```python
from build123d import *

# Parameters (mm, degrees)
F2_W     = 50
F2_H     = 40
F3_DEPTH = 1.5
F4_D     = 3.5


with BuildPart() as f3:
    # F2 (on Top) → F3 (new body)
    with BuildSketch(Plane.XY):
        Rectangle(F2_W, F2_H)
    extrude(amount=F3_DEPTH)

    # F4 (through all)
    with Locations(Plane(origin=(0, 0, 0), x_dir=(1, 0, 0), z_dir=(0, 0, -1))):
        with Locations((-22.2, 17.2), (-22.2, -17.2), (22.2, 17.2), (22.2, -17.2)):
            Hole(F4_D / 2)


solid = f3.part
```
The model under review builds one solid part; all positions refer to its coordinate system, in mm. Coordinates: 2 decimals unless noted, no trailing zeros. Write each loop counter-clockwise with the first axis right and the second up, starting at its lowest first coordinate (ties: lowest second). Pieces come first, ordered by that corner, then holes. Notation, with made-up numbers: (14.5, 8) - (49.5, 8) arc R27 cw to (49.5, 44) - close; hole circle Ø11 at (56, -29). An arc over 180 degrees is marked (long way). Write item = value, one per line.
(1) Consider section B-B, the plane y = -17.2. Give the boundary of the cut face in (x, z), then the cut area to 3 significant figures.
Result sheet:
outline = (-25, 0) - (-23.95, 0) - (-23.95, 1.5) - (-25, 1.5) - close; (-20.45, 0) - (20.45, 0) - (20.45, 1.5) - (-20.45, 1.5) - close; (23.95, 0) - (25, 0) - (25, 1.5) - (23.95, 1.5) - close
area = 64.5 mm^2
(2) For line 1 (X direction, y = -17.2, z = 0.9); line 2 (Y direction, x = -22.2, z = 0.7); line 3 (X direction, y = 16, z = 0.4), list the stretches that pass through material, from the lowest coordinate up. Write a range as [from, to].
Result sheet:
line_1 = [-25, -23.95], [-20.45, 20.45], [23.95, 25]
line_2 = [-20, -18.95], [-15.45, 15.45], [18.95, 20]
line_3 = [-25, -23.47], [-20.93, 20.93], [23.47, 25]
(3) Consider section C-C, the plane z = 0.8. Give the boundary of the cut face in (x, y), then the cut area to 3 significant figures.
Result sheet:
outline = (-25, -20) - (25, -20) - (25, 20) - (-25, 20) - close; hole circle Ø3.5 at (-22.2, -17.2); hole circle Ø3.5 at (-22.2, 17.2); hole circle Ø3.5 at (22.2, -17.2); hole circle Ø3.5 at (22.2, 17.2)
area = 1,960 mm^2
(4) Consider section A-A, the plane x = -22.2. Give the boundary of the cut face in (y, z), then the cut area to 3 significant figures.
Result sheet:
outline = (-20, 0) - (-18.95, 0) - (-18.95, 1.5) - (-20, 1.5) - close; (-15.45, 0) - (15.45, 0) - (15.45, 1.5) - (-15.45, 1.5) - close; (18.95, 0) - (20, 0) - (20, 1.5) - (18.95, 1.5) - close
area = 49.5 mm^2
(5) Mouldability with a two-part tool opening along X and no side actions: class faces 1 (the face through (0, -20, 1)), 2 (the face through (-25, 0, 1)), 3 (the face through (20.531, 16.674, 0.76)) as pulls with the +X half, pulls with the -X half, needs draft (parallel to the pull), parting line crosses it, or undercut.
Result sheet:
face_1 = needs draft
face_2 = pulls with the -X half
face_3 = undercut
